```python
from build123d import *

# Parameters (mm, degrees)
SKETCH2_W                = 20
SKETCH2_H                = 70
BOSS_EXTRUDE1_DEPTH      = 30
SKETCH3_R                = 4
CUT_EXTRUDE1_DEPTH       = 20
SKETCH4_R                = 2.5
CUT_EXTRUDE2_DEPTH       = 10
FILLET1_R                = 10
BOSS_EXTRUDE2_DEPTH      = 100
BOSS_EXTRUDE2_DEPTH_BACK = 40
SKETCH5_W                = 5
SKETCH5_H                = 30
SKETCH6_R                = 2.5
SKETCH6_W                = 100
SKETCH6_H                = 20
CUT_EXTRUDE3_DEPTH       = 5
FILLET2_R                = 5
CUT_EXTRUDE5_REACH       = 132.074
SKETCH8_W                = 6
SKETCH8_H                = 10


with BuildPart() as part:
    # Sketch2 → Boss-Extrude1 (new body)
    with BuildSketch(Plane(origin=(0, 0, 0), x_dir=(1, 0, 0), z_dir=(0, 1, 0))):
        with Locations((6.47761194, -5.23880597)):
            Rectangle(SKETCH2_W, SKETCH2_H)
    extrude(amount=BOSS_EXTRUDE1_DEPTH)

    # Sketch3 → Cut-Extrude1 (cut)
    with BuildSketch(Plane(origin=(0, 30, 0), x_dir=(1, 0, 0), z_dir=(0, 1, 0))):
        with Locations(Location((6.47761194, 19.26119403, 0), (0, 0, 270))):
            Circle(SKETCH3_R)
        with Locations(Location((6.47761194, -29.73880597, 0), (0, 0, 270))):
            Circle(SKETCH3_R)
    extrude(amount=-CUT_EXTRUDE1_DEPTH, mode=Mode.SUBTRACT)

    # Sketch4 → Cut-Extrude2 (cut)
    with BuildSketch(Plane.ZY.offset(3.52238806)):
        with BuildLine():
            Line((17.415034126, 30.126407987), (14.795699792, 30.126407987))
            Line((14.795699792, 30.126407987), (14.949961333, 28.969446425))
            ThreePointArc((14.949961333, 28.969446425), (16.17927412, 22.186618473), (17.347611009, 28.980215007))
            Line((17.347611009, 28.980215007), (17.415034126, 30.126407987))
        make_face()
        with Locations((16.163554702, 25.686583173)):
            Circle(SKETCH4_R, mode=Mode.SUBTRACT)
    extrude(amount=-CUT_EXTRUDE2_DEPTH, mode=Mode.SUBTRACT)

    # Fillet1
    fillet1_edges = [part.edges().sort_by_distance(p)[0] for p in [
        (-3.52238806, 15, -29.76119403),
        (16.47761194, 15, -29.76119403),
        (16.47761194, 15, 40.23880597),
        (-3.52238806, 15, 40.23880597),
    ]]
    fillet(fillet1_edges, radius=FILLET1_R - 0.0001)  # a hair under: the kernel refuses the full size

    # Sketch5 → Boss-Extrude2 (add, two sides: drawn at the far end of the back side and taken through both)
    with BuildSketch(Plane.ZY.offset(3.52238806).offset(-BOSS_EXTRUDE2_DEPTH_BACK)):
        with Locations((-1.26119403, 15)):
            Rectangle(SKETCH5_W, SKETCH5_H)
    extrude(amount=BOSS_EXTRUDE2_DEPTH + BOSS_EXTRUDE2_DEPTH_BACK)

    # Sketch6 → Cut-Extrude3 (cut)
    with BuildSketch(Plane(origin=(0, 0, -3.76119403), x_dir=(-1, 0, 0), z_dir=(0, 0, -1))):
        with Locations((-26.47761194, 5)):
            Circle(SKETCH6_R)
        with Locations((53.52238806, 20)):
            Rectangle(SKETCH6_W, SKETCH6_H)
        with BuildLine():
            Line((93.519935535, 2.406805213), (-1.480064465, 2.500001203))
            ThreePointArc((-1.480064465, 2.500001203), (-3.977610737, 5.002452525), (-1.475159415, 7.499998797))
            Line((-1.475159415, 7.499998797), (93.524840585, 7.406802807))
            ThreePointArc((93.524840585, 7.406802807), (96.022386857, 4.904351485), (93.519935535, 2.406805213))
        make_face()
    extrude(amount=-CUT_EXTRUDE3_DEPTH, mode=Mode.SUBTRACT)

    # Fillet2
    fillet2_edges = [part.edges().sort_by_distance(p)[0] for p in [
        (36.47761194, 30, -1.26119403),
        (36.47761194, 0, -1.26119403),
        (-103.52238806, 10, -1.26119403),
        (-103.52238806, 0, -1.26119403),
    ]]
    fillet(fillet2_edges, radius=FILLET2_R - 0.0001)  # a hair under: the kernel refuses the full size

    # Sketch8 → Cut-Extrude5 (cut, up to next)
    with BuildSketch(Plane(origin=(16.47761194, 0, 0), x_dir=(0, 0, -1), z_dir=(1, 0, 0)), mode=Mode.PRIVATE) as cut_extrude5_sk1:
        with Locations((6.76119403, 5)):
            Rectangle(SKETCH8_W, SKETCH8_H)
    cut_extrude5_tool1 = extrude(cut_extrude5_sk1.sketch, amount=-CUT_EXTRUDE5_REACH, mode=Mode.PRIVATE) & part.part
    add(cut_extrude5_tool1.solids().sort_by_distance((16.477612, 5, -6.761194))[0], mode=Mode.SUBTRACT)


solid = part.part
```
Read the model definition and answer for the solid it produces. Units are mm, in the model's axes. A direction names the side the tool comes from. Coordinates: 2 decimals unless noted, no trailing zeros. Write each loop counter-clockwise with the first axis right and the second up, starting at its lowest first coordinate (ties: lowest second). Pieces come first, ordered by that corner, then holes. Notation, with made-up numbers: (75.5, 25.5) -> (112.5, 25.5) arc R15 ccw to (112.5, 35.5) -> close; hole circle Ø11 at (28.25, -2.5). An arc over 180 degrees is marked (long way). Return JSON: item names as keys, results as strings.
1. A cutting plane is placed at C-C (z = 11). Determine the outline of the cut face in (x, y).
Found:
{"outline": "(-3.52, 0) -> (16.48, 0) -> (16.48, 30) -> (-3.52, 30) -> close"}
2. A cutting plane is placed at B-B (x = 26). Determine the outline of the cut face in (y, z), and give its area (3 significant figures).
Found:
{"outline": "(0, -3.76) -> (2.55, -3.76) -> (2.55, 1.24) -> (0, 1.24) -> close; (7.45, -3.76) -> (30, -3.76) -> (30, 1.24) -> (7.45, 1.24) -> close", "area": "125 mm2"}
3. Find the intervals of material crossed by line 1 along X through (y, z) = (1.5, -18); line 2 along Z through (x, y) = (9, 24); line 3 along Z through (x, y) = (7, 10.25), in increasing order. Write a range as from..to.
Found:
{"line 1": "-3.52..16.48", "line 2": "-29.44..-22.37, -16.16..26.63, 32.84..39.92", "line 3": "-29.75..-23.23, -15.3..25.77, 33.7..40.23"}
4. A cutting plane is placed at A-A (y = 14.75). Give the number of separate pieces and of enclosed holes in the cut face, and give its area (3 significant figures).
Found:
{"separate pieces": "1", "enclosed holes": "2", "area": "1,310 mm2"}
5. A cutting plane is placed at D-D (x = -2). Determine the outline of the cut face in (y, z).
Found:
{"outline": "(0, -25.07) -> (30, -25.07) -> (30, 14.81) -> (28.97, 14.95) arc R3.5 cw (long way) to (28.98, 17.35) -> (30, 17.41) -> (30, 35.54) -> (0, 35.54) -> (0, -3.76) -> (2.5, -3.76) -> (2.5, 1.24) -> (7.5, 1.24) -> (7.5, -3.76) -> (10, -3.76) -> (10, -9.76) -> (0, -9.76) -> close; circle Ø5 at (25.69, 16.16)"}
6. Each of these flat-tipped pins is pushed along its axis until it touches: P1, Ø8, axis at y = 20.5, z = -13.5, coming from the +X side; P2, Ø5.5, axis at x = -63, z = -1.5, coming from the +Y side; P3, Ø9, axis at x = 7, z = -21, coming from the +Y side; P4, Ø1.5, axis at y = 10, z = 23, coming from the -X side. Where does it stop, or does it pass through?
Found:
{"P1": "x = 16.48", "P2": "y = 10", "P3": "y = 30", "P4": "x = -3.52"}
7. A tool of negligible diameter and unlimited length cuts with its end or side. For faces 4 (the face through (-50, 10, -1)), 5 (the face through (16.478, 15, -12)), 6 (the face through (-12, 8, -3.761)), 7 (the face through (16.478, 15, 16)), 8 (the face through (7.679, 20.14, 33.554)), from which of +Z, -Z, +X, -X, +Y, -Y can it reach the whole face along a straight path? Write none if from no direction.
Found:
{"face 4": "+Z, -Z, -X, +Y", "face 5": "-Z, +X, +Y, -Y", "face 6": "+X, -Y", "face 7": "+Z, +X, +Y, -Y", "face 8": "+Y"}
8. Determine the mould class of faces 1 (the face through (7, 0, -20)), 2 (the face through (7, 10, -7)), 3 (the face through (-0.7, 15.2, 37.2)) for opening direction Z: pulls with the +Z half, pulls with the -Z half, needs draft (parallel to the pull), parting line crosses it, or undercut.
Found:
{"face 1": "needs draft", "face 2": "undercut", "face 3": "pulls with the +Z half"}
